Geometry check sheet. Reference: the model listing, model coordinates, mm. A direction names the side the tool comes from. Coordinates: 2 decimals unless noted, no trailing zeros. Loops run counter-clockwise (first coordinate to the right, second up) from the corner with the lowest first, then second, coordinate; pieces in that order, holes last. Notation, with made-up numbers: (10.5, 78) - (63.5, 78) arc R30 ccw to (63.5, 107) - close; hole circle Ø5 at (45.25, 42.25). An arc over 180 degrees is marked (long way). One line per item, written item: value.
Autodesk Inventor part; units mm, degrees
ref_plane "YZ Plane" through (0, 0, 0) normal (1, 0, 0) x (0, 1, 0)
ref_plane "XZ Plane" through (0, 0, 0) normal (0, 1, 0) x (-1, 0, 0)
ref_plane "XY Plane" through (0, 0, 0) normal (0, 0, 1) x (1, 0, 0)
sketch "Sketch1" plane through (0, 0, 0) normal (0, 0, 1) x (1, 0, 0)
  line L0 (125.272, 1.0352) -> (94.9914, -14.9276)
  arc A0 (97.3229, -19.3507) -> (94.9914, -14.9276) centre (89.9019, -20.4364) ccw
  line L1 (97.3229, -19.3507) -> (127.6037, -3.3892)
  line L2 (157.89, 12.5592) -> (127.6037, -3.3892)
  arc A1 (155.5603, 16.9833) -> (157.89, 12.5592) centre (162.9818, 18.0659) ccw
  line L3 (125.272, 1.0352) -> (155.5603, 16.9833)
  circle A2 centre (162.9818, 18.0659) radius 4.5
  circle A3 centre (162.9818, 18.0659) radius 7.5
  arc A4 (192.0328, 98.1186) -> (196.6808, 96.2757) centre (196.9631, 103.7704) ccw
  line L4 (163.264, 25.5606) -> (192.0328, 98.1186)
  arc A5 (167.912, 23.7177) -> (163.264, 25.5606) centre (162.9818, 18.0659) ccw
  line L5 (196.6808, 96.2757) -> (167.912, 23.7177)
  circle A6 centre (196.9631, 103.7704) radius 4.5
  circle A7 centre (196.9631, 103.7704) radius 7.5
  circle A8 centre (89.9019, -20.4364) radius 4.5
  circle A9 centre (89.9019, -20.4364) radius 7.5
  arc A10 (6.341, -4.0052) -> (7.4493, 0.8704) centre (0, 0) ccw
  line L6 (6.341, -4.0052) -> (82.4526, -21.3068)
  arc A11 (83.5609, -16.4312) -> (82.4526, -21.3068) centre (89.9019, -20.4364) ccw
  line L7 (83.5609, -16.4312) -> (7.4493, 0.8704)
  circle A12 centre (0, 0) radius 4.5
  circle A13 centre (0, 0) radius 7.5
  circle A14 centre (105.6859, 38.2113) radius 3.464 construction
  circle A15 centre (101.9441, 45.313) radius 4.5 construction
  arc A16 (109.4545, 45.313) -> (97.6972, 39.1186) centre (101.9441, 45.313) ccw construction
  circle A17 centre (105.6859, 38.2113) radius 4.5
  line L8 (111.3563, 33.3025) -> (155.487, 17.786)
  arc A18 (106.528, 30.7587) -> (111.3563, 33.3025) centre (105.6859, 38.2113) ccw
  arc A19 (113.1807, 38.4912) -> (101.217, 32.1881) centre (105.6859, 38.2113) ccw
  line L9 (157.3113, 22.9747) -> (113.1807, 38.4912)
  line L10 (163.0842, 20.9449) -> (163.0574, 20.9543)
  line L11 (101.217, 32.1881) -> (89.0598, -12.9838)
  line L12 (94.3708, -14.4132) -> (106.528, 30.7587)
  point P0 (0, 0)
  point P1 (97.7939, 8.8875)
  point P2 (134.3338, 28.1386)
  dimension "d0" = 9
  dimension "d2" = 7.5104
  dimension "d5" = 0.002
extrude "Extrusion1" add sketch "Sketch1" along normal blind 4 contours A0 A9 | A3 A1 | A9 L11 A19 L9 A3 L8 A18 L12 | L6 A10 L7 A9 | A3 L4 A4 L5 | A13 A10 | A4 A7
sketch "Sketch2" plane through (0, 0, 4) normal (0, 0, 1) x (1, 0, 0)
  circle A0 centre (0, 0) radius 4.5
  circle A1 centre (0, 0) radius 7.5
  circle A2 centre (196.9631, 103.7704) radius 4.5
  circle A3 centre (196.9631, 103.7704) radius 4.5
  circle A4 centre (196.9631, 103.7704) radius 7.5
extrude "Extrusion2" add sketch "Sketch2" along normal blind 9
sketch "Sketch3" plane through (0, 0, 4) normal (0, 0, 1) x (1, 0, 0)
  circle A0 centre (89.9019, -20.4364) radius 4.5
  circle A1 centre (89.9019, -20.4364) radius 4.5
  circle A2 centre (89.9019, -20.4364) radius 7.5
  circle A3 centre (105.6859, 38.2113) radius 4.5
  circle A4 centre (105.6859, 38.2113) radius 4.5
  circle A5 centre (105.6859, 38.2113) radius 7.5
  circle A6 centre (162.9818, 18.0659) radius 4.5
  circle A7 centre (162.9818, 18.0659) radius 4.5
  circle A8 centre (162.9818, 18.0659) radius 7.5
  point P0 (0, 0)
extrude "Extrusion3" add sketch "Sketch3" along normal blind 1
scale "Scale1" factors (0.5, 0.5, 0.5) then translate (55.6782, 16.6513, 0) bodies 1
properties part number "MassiveGearHOlder"
(1) Material ranges on probe 1 along X at (y, z) = (69, 3.25); probe 2 along X at (y, z) = (49.5, 1.5); probe 3 along X at (y, z) = (19, 4), recorded low to high. Write a range as from..to.
Reply:
probe 1: 150.44..151.96, 156.36..157.88
probe 2: 145.27..147.96
probe 3: 52.75..58.6
(2) Cross-section at A-A on z = 4. Record the cut outline in (x, y), and give its area (3 significant figures).
Reply:
outline: circle Ø7.5 at (55.68, 16.65); circle Ø7.5 at (154.16, 68.54); hole circle Ø4.5 at (55.68, 16.65); hole circle Ø4.5 at (154.16, 68.54)
area: 56.5 mm2
(3) Go/stop test with flat-tipped pins: pin 1 Ø8.5 at (x, y) = (125, 33) entering from +Z; pin 2 Ø1.5 at (y, z) = (16.5, 4) entering from +X; pin 3 Ø2 at (x, z) = (66, 2) entering from -Y. Record where each tip stops, or that it passes through.
Reply:
pin 1: z = 2
pin 2: x = 59.43
pin 3: y = 12.8
(4) Release check for a two-part mould opening along X. For faces 4 (the face through (139, 24, 2.5)), 5 (the face through (77.61, 10.384, 0.986)) record: pulls with the +X half, pulls with the -X half, needs draft (parallel to the pull), parting line crosses it, or undercut.
Reply:
face 4: needs draft
face 5: undercut
(5) Cross-section at C-C on x = 125.5. Record the cut outline in (y, z), and give its area (3 significant figures).
Reply:
outline: (28.33, 0) - (31.24, 0) - (31.24, 2) - (28.33, 2) - close
area: 5.83 mm2
(6) Access from +Z, -Z, +X, -X, +Y, -Y to the whole of each face (thin tool, end or side, straight path). Record for faces 1 (the face through (110.29, 32.45, 0.99)), 2 (the face through (123.46, 31.96, 0.99)), 3 (the face through (103.29, 21.61, 0.99)).
Reply:
face 1: +Z, -Z, -Y
face 2: +Z, -Z, +Y
face 3: +Z, -Z
(7) Cross-section at B-B on y = 62. Record the cut outline in (x, z), and give its area (3 significant figures).
Reply:
outline: (150.22, 0) - (152.91, 0) - (152.91, 2) - (150.22, 2) - close
area: 5.38 mm2
